Source: CAD feature listing. Evaluate the final solid. Frame: model axes, mm. A direction names the side the tool comes from. Round coordinates to 2 decimals unless told otherwise and drop trailing zeros. Write each loop counter-clockwise with the first axis right and the second up, starting at its lowest first coordinate (ties: lowest second). Pieces come first, ordered by that corner, then holes. Notation, with made-up numbers: M 6,61 L 57,61 A10 cw 57,69 Z; hole C 77,3.25 d7. An arc over 180 degrees is marked long. Answer in a Markdown table with one row per item.
from build123d import *

# Parameters (mm, degrees)
SKETCH_1_R          = 11.95
EXTRUDE_1_DEPTH     = 10.23
SKETCH_2_R          = 7
CUT_EXTRUDE_1_DEPTH = 20.754946216
CHAMFER_1_SIZE      = 2.15
SKETCH_3_R          = 8
CUT_EXTRUDE_2_DEPTH = 4.515
CHAMFER_2_SIZE      = 0.8


with BuildPart() as part:
    # Эскиз1 → Бобышка-Вытянуть1 (new body)
    with BuildSketch(Plane.XY):
        Circle(SKETCH_1_R)
    extrude(amount=EXTRUDE_1_DEPTH)

    # Эскиз2 → Вырез-Вытянуть1 (cut, through all)
    with BuildSketch(Plane.XY.offset(10.23)):
        Circle(SKETCH_2_R)
    extrude(amount=-CUT_EXTRUDE_1_DEPTH, mode=Mode.SUBTRACT)

    # Фаска1
    chamfer_1_edges = [part.edges().sort_by_distance(p)[0] for p in [
        (-11.95, 0, 0),
        (-11.95, 0, 10.23),
    ]]
    chamfer(chamfer_1_edges, length=CHAMFER_1_SIZE)

    # Эскиз3 → Вырез-Вытянуть2 (cut)
    with BuildSketch(Plane.XY.offset(10.23)):
        Circle(SKETCH_3_R)
    cut_extrude_2 = extrude(amount=-CUT_EXTRUDE_2_DEPTH, mode=Mode.SUBTRACT)

    # Зеркальное отражение1: Вырез-Вытянуть2 across plane
    add(cut_extrude_2.mirror(Plane(origin=(0, 0, 5.115), x_dir=(1, 0, 0), z_dir=(0, 0, -1))), mode=Mode.SUBTRACT)

    # Фаска2
    chamfer_2_edges = [part.edges().sort_by_distance(p)[0] for p in [
        (-8, 0, 10.23),
        (-8, 0, 0),
    ]]
    chamfer(chamfer_2_edges, length=CHAMFER_2_SIZE)


solid = part.part
Q1. Section D-D (z = 9.75). Return loops of the section in (x, y), and give its area (3 significant figures).
Solutions:
| item | result |
|---|---|
| outline | C 0,0 d20.56; hole C 0,0 d16.64 |
| area | 115 mm2 |
Q2. Section A-A (x = 0). Return loops of the section in (y, z) (3 decimals).
Solutions:
| item | result |
|---|---|
| outline | M -11.95,2.15 L -9.8,0 L -8.8,0 L -8,0.8 L -8,4.515 L -7,4.515 L -7,5.715 L -8,5.715 L -8,9.43 L -8.8,10.23 L -9.8,10.23 L -11.95,8.08 Z; M 7,4.515 L 8,4.515 L 8,0.8 L 8.8,0 L 9.8,0 L 11.95,2.15 L 11.95,8.08 L 9.8,10.23 L 8.8,10.23 L 8,9.43 L 8,5.715 L 7,5.715 Z |
Q3. Pull-direction query (Y, two-part tool) for faces 1 (the cylindrical face through (-1.73, -7.81, 7.6)), 2 (the flat face through (-7, 6, 10.23)), 3 (the conical face through (4.6, -8.8, 10.1)); classes: pulls with the +Y half, pulls with the -Y half, needs draft (parallel to the pull), parting line crosses it, or undercut.
Solutions:
| item | result |
|---|---|
| face 1 | undercut |
| face 2 | needs draft |
| face 3 | parting line crosses it |
Q4. Contact query for flat-ended pins moving along their axis: pin 1 Ø9.5 at (x, y) = (0, 0) entering from +Z; pin 2 Ø1 at (x, z) = (4, 2.5) entering from +Y; pin 3 Ø1.5 at (y, z) = (-0.5, 2) entering from +X; pin 4 Ø2 at (x, z) = (-2.5, 4.5) entering from +Y. Output: stop coordinate, or through.
Solutions:
| item | result |
|---|---|
| pin 1 | passes through |
| pin 2 | stops at y = 11.43 |
| pin 3 | stops at x = 11.95 |
| pin 4 | stops at y = 11.86 |
Q5. Section C-C (z = 5). Return loops of the section in (x, y).
Solutions:
| item | result |
|---|---|
| outline | C 0,0 d23.9; hole C 0,0 d14 |
Q6. Material intervals for probe 1 along Y at (x, z) = (0, 5.3); probe 2 along X at (y, z) = (4.5, 9.25); probe 3 along Z at (x, y) = (-2.5, 7) (3 decimals), sorted ascending.
Solutions:
| item | result |
|---|---|
| probe 1 | y = -11.95 to -7, 7 to 11.95 |
| probe 2 | x = -9.8 to -6.61, 6.61 to 9.8 |
| probe 3 | z = 4.515 to 5.715 |
Q7. Access query for faces 4 (the flat face through (4, -6, 4.515)), 5 (the flat face through (4, -6, 5.715)), 6 (the cylindrical face through (6.42, 10.08, 5.07)). Directions: +Z, -Z, +X, -X, +Y, -Y. A direction counts if a zero-diameter tool reaches every point of the face in a straight line with its end or side. Return the directions, or none.
Solutions:
| item | result |
|---|---|
| face 4 | -Z |
| face 5 | +Z |
| face 6 | +Z, -Z |
